Autodesk Inventor part; units mm, degrees
ref_plane "YZ Plane" through (0, 0, 0) normal (1, 0, 0) x (0, 1, 0)
ref_plane "XZ Plane" through (0, 0, 0) normal (0, 1, 0) x (-1, 0, 0)
ref_plane "XY Plane" through (0, 0, 0) normal (0, 0, 1) x (1, 0, 0)
sketch "Sketch1" plane through (0, 0, 0) normal (1, 0, 0) x (0, 1, 0)
  line L0 (7.6752, 16.382) -> (7.6752, -31.243)
  line L1 (7.6752, 16.382) -> (7.6752, 64.007)
  line L2 (-2.4848, 16.382) -> (-2.4848, 64.007)
  line L3 (0.6902, 67.182) -> (4.5002, 67.182)
  line L4 (-2.4848, 16.382) -> (-2.4848, -31.243)
  line L5 (0.6902, -34.418) -> (4.5002, -34.418)
  arc A0 (7.6752, 64.007) -> (4.5002, 67.182) centre (4.5002, 64.007) ccw
  arc A1 (4.5002, -34.418) -> (7.6752, -31.243) centre (4.5002, -31.243) ccw
  line L6 (-2.4848, 64.007) -> (-2.4848, 67.182)
  line L7 (-2.4848, 67.182) -> (0.6902, 67.182)
  line L8 (-2.4848, -31.243) -> (-2.4848, -34.418)
  line L9 (0.6902, -34.418) -> (-2.4848, -34.418)
  circle A2 centre (2.5952, 16.382) radius 4
  point P0 (0, 0)
  point P1 (7.6752, -34.418)
  point P2 (7.6752, 67.182)
  dimension "d1" = 50.8
  dimension "d2" = 50.8
  dimension "d3" = 3.175
  dimension "d101" = 8
extrude "Extrusion1" add sketch "Sketch1" along normal blind 1.27 contours L0 A1 L5 L9 L8 L4 L2 L6 L7 L3 A0 L1 | A2
sketch "Sketch4" plane through (0, -2.4848, 16.382) normal (0, -1, 0) x (1, 0, 0)
  line L0 (1.27, 50.8) -> (1.27, -50.8)
  line L1 (1.27, 0) -> (1.27, 47.625)
  line L2 (0.9525, 50.8) -> (0.9525, 25.4)
  line L3 (0.9525, 50.8) -> (0.3175, 50.8)
  line L4 (0.3175, 50.8) -> (0.3175, 25.4)
  line L5 (0.3175, 25.4) -> (0.9525, 25.4)
  line L6 (0, -50.8) -> (1.27, -50.8)
  line L7 (0.9525, -50.8) -> (0.9525, -25.4)
  line L8 (0.9525, -25.4) -> (0.3175, -25.4)
  line L9 (0.3175, -25.4) -> (0.3175, -50.8)
  line L10 (0.9525, -50.8) -> (0.3175, -50.8)
  point P0 (0, -16.382)
  dimension "d27" = 25.4
  dimension "d28" = 0.635
  dimension "d29" = 25.4
  dimension "d31" = 25.4
  dimension "d32" = 0.635
extrude "Extrusion3" add sketch "Sketch4" along normal blind 106.68
sketch "Sketch5" plane through (0.9525, -2.4848, 67.182) normal (1, 0, 0) x (0, 0, -1)
  line L0 (0, 6.985) -> (0, 0)
  line L1 (0, 0) -> (0, -106.68)
  line L2 (25.4, 0) -> (25.4, -106.68)
  line L3 (0, 0) -> (101.6, 0)
  line L4 (6.985, -3.81) -> (18.415, -3.81)
  line L5 (21.59, -6.985) -> (21.59, -99.695)
  line L6 (18.415, -102.87) -> (6.985, -102.87)
  line L7 (3.81, -99.695) -> (3.81, -6.985)
  line L8 (25.4, -106.68) -> (0, -106.68)
  arc A0 (6.985, -3.81) -> (3.81, -6.985) centre (6.985, -6.985) ccw
  arc A1 (21.59, -6.985) -> (18.415, -3.81) centre (18.415, -6.985) ccw
  arc A2 (3.81, -99.695) -> (6.985, -102.87) centre (6.985, -99.695) ccw
  arc A3 (18.415, -102.87) -> (21.59, -99.695) centre (18.415, -99.695) ccw
  line L9 (83.185, -3.81) -> (94.615, -3.81)
  line L10 (97.79, -6.985) -> (97.79, -99.695)
  line L11 (94.615, -102.87) -> (83.185, -102.87)
  line L12 (80.01, -99.695) -> (80.01, -6.985)
  line L13 (101.6, 0) -> (101.6, -106.68)
  line L14 (50.8, 0) -> (101.6, 0)
  line L15 (76.2, 0) -> (76.2, -106.68)
  line L16 (101.6, -106.68) -> (76.2, -106.68)
  arc A4 (83.185, -3.81) -> (80.01, -6.985) centre (83.185, -6.985) ccw
  arc A5 (97.79, -6.985) -> (94.615, -3.81) centre (94.615, -6.985) ccw
  arc A6 (80.01, -99.695) -> (83.185, -102.87) centre (83.185, -99.695) ccw
  arc A7 (94.615, -102.87) -> (97.79, -99.695) centre (94.615, -99.695) ccw
  point P0 (67.182, 2.4848)
  dimension "d67" = 3.81
  dimension "d68" = 3.81
  dimension "d69" = 3.81
  dimension "d70" = 3.81
  dimension "d71" = 3.175
  dimension "d72" = 3.81
  dimension "d73" = 3.81
  dimension "d74" = 3.81
  dimension "d75" = 3.81
  dimension "d76" = 3.175
extrude "Extrusion5" cut sketch "Sketch5" against normal through all contours L4 A1 L5 A3 L6 A2 L7 A0 | L9 A5 L10 A7 L11 A6 L12 A4
sketch "Sketch6" plane through (1.27, 0, 0) normal (1, 0, 0) x (0, 0, -1)
  line L0 (-67.182, -2.4848) -> (34.418, -2.4848)
  line L1 (-16.382, 7.6752) -> (-64.007, 7.6752)
  line L2 (-41.782, -2.4848) -> (-67.182, -2.4848)
  arc A0 (-64.007, 4.1192) -> (-64.007, 1.0712) centre (-64.007, 2.5952) ccw
  arc A1 (-16.382, 7.6752) -> (-16.382, -2.4848) centre (-16.382, 2.5952) ccw
  arc A2 (-24.637, 1.0712) -> (-24.637, 4.1192) centre (-24.637, 2.5952) ccw
  line L3 (-64.007, 4.1192) -> (-24.637, 4.1192)
  line L4 (-64.007, 1.0712) -> (-24.637, 1.0712)
  point P0 (0, 0)
  dimension "d90" = 3.048
extrude "Extrusion6" cut sketch "Sketch6" against normal through all
sketch "Sketch7" plane through (1.27, 0, 0) normal (1, 0, 0) x (0, 0, -1)
  arc A0 (-16.382, -2.4848) -> (-16.382, 7.6752) centre (-16.382, 2.5952) ccw
  arc A1 (-8.127, 4.1192) -> (-8.127, 1.0712) centre (-8.127, 2.5952) ccw
  arc A2 (31.2702, 1.0712) -> (31.2702, 4.1192) centre (31.2702, 2.5952) ccw
  line L0 (31.2702, 4.1192) -> (-8.127, 4.1192)
  line L1 (-8.127, 1.0712) -> (31.2702, 1.0712)
  point P0 (0, 0)
  dimension "d96" = 3.048
  dimension "d98" = 3.048
extrude "Extrusion7" cut sketch "Sketch7" against normal through all
sketch "Sketch8" plane through (1.27, 0, 0) normal (1, 0, 0) x (0, 0, -1)
  arc A0 (-24.637, 1.0712) -> (-24.637, 4.1192) centre (-24.637, 2.5952) ccw
  circle A1 centre (-16.382, 2.5952) radius 4
  point P0 (0, 0)
  dimension "d103" = 8
extrude "Extrusion8" cut sketch "Sketch8" against normal through all
properties part number "Part On Monitor"
Verification items for the finished model (mm, model axes). A direction names the side the tool comes from. Give positions to 0.01 mm unless a question says otherwise; leave off trailing zeros. Order: outer loops, then holes, each group sorted by start corner. A loop starts at its lowest first (then second) coordinate and runs counter-clockwise, first axis right, second up. Notation, with made-up numbers: (-32, -30) -> (22, -30) arc R25 ccw to (22, 6) -> close; hole circle Ø3 at (4, 15.25). An arc over 180 degrees is marked (long way). One line per item, written item: value.
(1) Gauge pin test, flat end, axial feed: pin 1 (3 mm diameter, centred on y = -46, z = -12.5, fed in from +X). Record the tip position at first contact, or that the pin passes through.
Final values:
pin 1: x = 0.95
(2) Tool access check on faces 4 (the face through (0.952, -60, -31)), 5 (the face through (0.318, -60, -12)), 6 (the face through (0.639, -104.4, 62.467)). Record the directions out of +Z, -Z, +X, -X, +Y, -Y that give a thin tool (end or side, any length) a straight path to the whole face; none if there is none.
Final values:
face 4: +Z, -Z, +X, -Y
face 5: +Z, -Z, -X, -Y
face 6: +X, -X
(3) Scan lines: line 1 along Z through (x, y) = (0.7, -53); line 2 along Y through (x, z) = (0.65, -26.5); line 3 along Y through (x, z) = (0.1, 42.5). Record each from-to range of solid material in increasing order. Write a range as [from, to].
Final values:
line 1: [-34.42, -30.61], [-12.83, -9.02], [41.78, 45.59], [63.37, 67.18]
line 2: [-109.16, -105.35], [-6.29, 1.07], [4.12, 7.68]
line 3: [-2.48, 1.07], [4.12, 7.68]
(4) Sectioned sample at A-A on y = -81.5. Record the cut outline in (x, z), then the cut area to 3 significant figures.
Final values:
outline: (0.32, -34.42) -> (0.95, -34.42) -> (0.95, -30.61) -> (0.32, -30.61) -> close; (0.32, -12.83) -> (0.95, -12.83) -> (0.95, -9.02) -> (0.32, -9.02) -> close; (0.32, 41.78) -> (0.95, 41.78) -> (0.95, 45.59) -> (0.32, 45.59) -> close; (0.32, 63.37) -> (0.95, 63.37) -> (0.95, 67.18) -> (0.32, 67.18) -> close
area: 9.68 mm^2
(5) Sectioned sample at D-D on z = 54.5. Record the cut outline in (x, y).
Final values:
outline: (0, -2.48) -> (0.32, -2.48) -> (0.32, -6.29) -> (0.95, -6.29) -> (0.95, -2.48) -> (1.27, -2.48) -> (1.27, 1.07) -> (0, 1.07) -> close; (0, 4.12) -> (1.27, 4.12) -> (1.27, 7.68) -> (0, 7.68) -> close; (0.32, -109.16) -> (0.95, -109.16) -> (0.95, -105.35) -> (0.32, -105.35) -> close
(6) Sectioned sample at C-C on z = -14.5. Record the cut outline in (x, y).
Final values:
outline: (0, -2.48) -> (0.32, -2.48) -> (0.32, -6.67) -> (0.95, -6.67) -> (0.95, -2.48) -> (1.27, -2.48) -> (1.27, 1.07) -> (0, 1.07) -> close; (0, 4.12) -> (1.27, 4.12) -> (1.27, 7.68) -> (0, 7.68) -> close; (0.32, -109.16) -> (0.95, -109.16) -> (0.95, -104.98) -> (0.32, -104.98) -> close
(7) Draft check along Y on faces 1 (the face through (0.644, 0.161, 19.556)), 2 (the face through (0.626, 6.77, -33.463)), 3 (the face through (0.318, -60, 64)). Enter one of: pulls with the +Y half, pulls with the -Y half, needs draft (parallel to the pull), parting line crosses it, or undercut.
Final values:
face 1: undercut
face 2: pulls with the +Y half
face 3: needs draft
(8) Sectioned sample at B-B on z = -2. Record the cut outline in (x, y).
Final values:
outline: (0, -2.48) -> (1.27, -2.48) -> (1.27, 1.07) -> (0, 1.07) -> close; (0, 4.12) -> (1.27, 4.12) -> (1.27, 7.68) -> (0, 7.68) -> close
